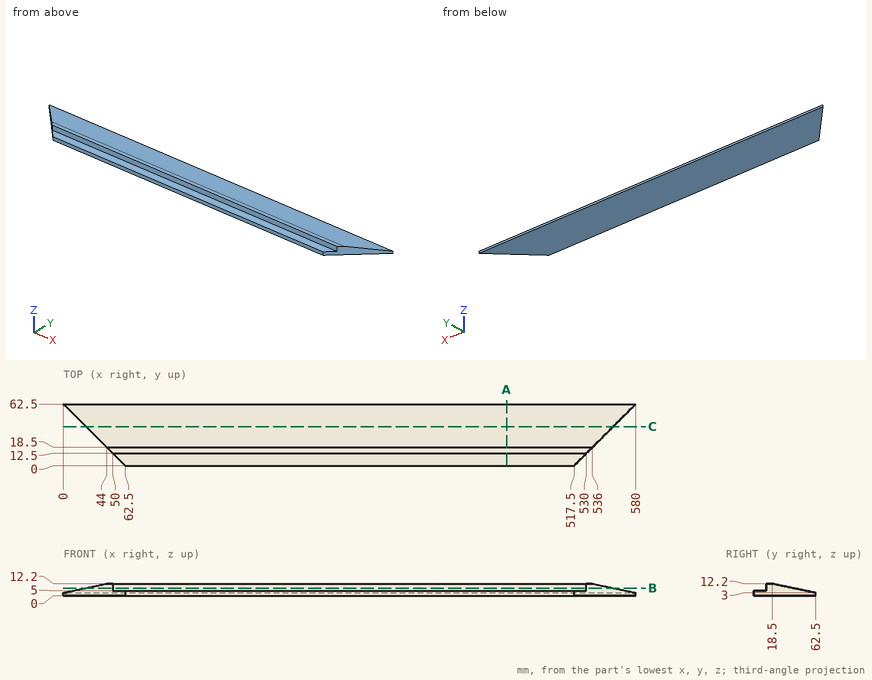
Here's the drawing with two shaded views (mm, measured from the low corner). I have some questions. Coordinates: 2 decimals unless noted, no trailing zeros. Order: outer loops, then holes, each group sorted by start corner. A loop starts at its lowest first (then second) coordinate and runs counter-clockwise, first axis right, second up. Notation, with made-up numbers: M 26,-6.5 L 38,-6.5 A13 cw 38,4.5 Z; hole C 47,69 d11. An arc over 180 degrees is marked long. Answer as CSV lines item,"result".
Item 1: Imagine slicing it at A-A on x = 449. Write out the boundary of the cut face in (y, z), plus the area to 3 significant figures.
Results found:
outline,"M 0,0 L 62.5,0 L 62.5,3 L 18.5,12.2 L 12.5,12.2 L 12.5,5 L 0,5 Z"
area,"470 mm2"
Item 2: For pin 1 (2 mm diameter, centred on x = 424.5, y = 22, fed in from -Z); pin 2 (1 mm diameter, centred on y = 42, z = 4.5, fed in from -X); pin 3 (10 mm diameter, centred on x = 319.5, y = 4.5, fed in from +Z); pin 4 (1.5 mm diameter, centred on y = 47.5, z = 7, fed in from -X), each with a flat end and sliding along its axis, tell me the tip position at first contact or that it passes through.
Results found:
pin 1,"z = 0"
pin 2,"x = 20"
pin 3,"z = 5"
pin 4,"through"
Item 3: Imagine slicing it at B-B on z = 7.75. Write out the boundary of the cut face in (x, y), plus the area to 3 significant figures.
Results found:
outline,"M 22.72,39.78 L 50,12.5 L 530,12.5 L 557.28,39.78 Z"
area,"13,800 mm2"
Item 4: If I drill on line 1 (Z direction, x = 143, y = 4.5); line 2 (Z direction, x = 298, y = 44); line 3 (X direction, y = 34, z = 3.5), over which ranges is the centre line in solid material (lowest first)?
Results found:
line 1,"0 to 5"
line 2,"0 to 6.87"
line 3,"28.5 to 551.5"
Item 5: Imagine slicing it at C-C on y = 39.5. Write out the boundary of the cut face in (x, z), plus the area to 3 significant figures.
Results found:
outline,"M 23,0 L 557,0 L 557,7.81 L 23,7.81 Z"
area,"4,170 mm2"
